Part model, mm, in its own coordinate system. A direction names the side the tool comes from. Round coordinates to 2 decimals unless told otherwise and drop trailing zeros. Write each loop counter-clockwise with the first axis right and the second up, starting at its lowest first coordinate (ties: lowest second). Pieces come first, ordered by that corner, then holes.
```python
from build123d import *

# Parameters (mm, degrees)
BOSS_EXTRUDE1_DEPTH = 18
SKETCH2_W           = 68
SKETCH2_H           = 20
CUT_EXTRUDE1_DEPTH  = 2
FILLET1_R           = 2
SKETCH3_W           = 20
SKETCH3_H           = 20
CUT_EXTRUDE4_DEPTH  = 7
SKETCH6_R           = 6.203606153
CUT_EXTRUDE5_DEPTH  = 103.004901843
CUT_EXTRUDE6_START  = -41
CUT_EXTRUDE6_DEPTH  = 41
FILLET2_R           = 6


# Read off the part's stored shape, not the designer's step: Cut-Extrude6
with BuildPart() as part:
    # Sketch1 → Boss-Extrude1 (new, symmetric)
    with BuildSketch(Plane.XY):
        with BuildLine():
            Line((-84, 0), (84, 0))
            Line((84, 0), (80, 14))
            Line((80, 14), (43, 14))
            Line((43, 14), (43, 55))
            Line((43, 55), (22, 55))
            Line((22, 55), (22, 43))
            Line((22, 43), (19, 43))
            Line((19, 43), (19, 40))
            ThreePointArc((19, 40), (0, 21), (-19, 40))
            Line((-19, 40), (-19, 43))
            Line((-19, 43), (-22, 43))
            Line((-22, 43), (-22, 55))
            Line((-22, 55), (-43, 55))
            Line((-43, 55), (-43, 14))
            Line((-43, 14), (-80, 14))
            Line((-80, 14), (-84, 0))
        make_face()
    extrude(amount=BOSS_EXTRUDE1_DEPTH, both=True)

    # Sketch2 → Cut-Extrude1 (cut)
    with BuildSketch(Plane.XZ):
        with Locations((-42, 0)):
            Rectangle(SKETCH2_W, SKETCH2_H)
        with Locations((42, 0)):
            Rectangle(SKETCH2_W, SKETCH2_H)
    extrude(amount=-CUT_EXTRUDE1_DEPTH, mode=Mode.SUBTRACT)

    # Fillet1
    fillet1_edges = [part.edges().sort_by_distance(p)[0] for p in [
        (76, 2, 0),
        (8, 2, 0),
        (-8, 2, 0),
        (-76, 2, 0),
    ]]
    fillet(fillet1_edges, radius=FILLET1_R - 0.0001)  # a hair under: the kernel refuses the full size

    # Sketch3 → Cut-Extrude4 (cut)
    with BuildSketch(Plane.XZ):
        with Locations((-31, 0)):
            Rectangle(SKETCH3_W, SKETCH3_H)
        with Locations((31, 0)):
            Rectangle(SKETCH3_W, SKETCH3_H)
    extrude(amount=-CUT_EXTRUDE4_DEPTH, mode=Mode.SUBTRACT)

    # Sketch6 → Cut-Extrude5 (cut, through all)
    with BuildSketch(Plane.XZ):
        with Locations(Location((-31, 0, 0), (0, 0, 270))):
            Circle(SKETCH6_R)
        with Locations(Location((31, 0, 0), (0, 0, 90))):
            Circle(SKETCH6_R)
        with BuildLine():
            Line((-68, 5), (-60, 5))
            ThreePointArc((-60, 5), (-55, 0), (-60, -5))
            Line((-60, -5), (-68, -5))
            ThreePointArc((-68, -5), (-73, 0), (-68, 5))
        make_face()
        with BuildLine():
            Line((68, 5), (60, 5))
            ThreePointArc((60, 5), (55, 0), (60, -5))
            Line((60, -5), (68, -5))
            ThreePointArc((68, -5), (73, 0), (68, 5))
        make_face()
    extrude(amount=-CUT_EXTRUDE5_DEPTH, mode=Mode.SUBTRACT)

    # Cut-Extrude6 outline → Cut-Extrude6 (cut)
    with BuildSketch(Plane(origin=(0, 55, 0), x_dir=(1, 0, 0), z_dir=(0, 1, 0)).offset(CUT_EXTRUDE6_START)):
        with BuildLine():
            ThreePointArc((43, 0), (42.001212365, -9.214019744), (39.05124838, -18))
            Line((39.05124838, -18), (43, -18))
            Line((43, -18), (43, 0))
        make_face()
        with BuildLine():
            ThreePointArc((39.05124838, 18), (42.001212365, 9.214019744), (43, 0))
            Line((43, 0), (43, 18))
            Line((43, 18), (39.05124838, 18))
        make_face()
        with BuildLine():
            Line((-43, -18), (-39.05124838, -18))
            ThreePointArc((-39.05124838, -18), (-42.001212365, -9.214019744), (-43, 0))
            Line((-43, 0), (-43, -18))
        make_face()
        with BuildLine():
            Line((-43, 18), (-43, 0))
            ThreePointArc((-43, 0), (-42.001212365, 9.214019744), (-39.05124838, 18))
            Line((-39.05124838, 18), (-43, 18))
        make_face()
    extrude(amount=CUT_EXTRUDE6_DEPTH, mode=Mode.SUBTRACT)

    # Fillet2
    fillet2_edges = [part.edges().sort_by_distance(p)[0] for p in [
        (42.001212365, 14, -9.214019744),
        (-42.001212365, 14, 9.214019744),
    ]]
    fillet(fillet2_edges, radius=FILLET2_R)

    # Sketch8 → Cut-Revolve1 (revolve, cut)
    with BuildSketch(Plane.XY, mode=Mode.PRIVATE) as cut_revolve1_sk:
        Polygon((0, 21), (0, 13.435755104), (3, 15.238336961), (3, 21.238336961), align=None)
    revolve(cut_revolve1_sk.sketch.rotate(Axis((0, 21, 0), (0, -1, 0)), 180), axis=Axis((0, 21, 0), (0, -1, 0)), mode=Mode.SUBTRACT)


solid = part.part
```
Q1. Drop flat-ended pins along their axis: pin 1 (1 mm diameter, centred on x = 11.5, z = -12.5, fed in from +Y); pin 2 (4 mm diameter, centred on x = 35.5, z = -5, fed in from -Y); pin 3 (3.5 mm diameter, centred on x = -16, z = -2.5, fed in from -Y). Give the stop position or say it passes through.
Values follow:
pin 1: stops at y = 25.27
pin 2: stops at y = 7
pin 3: stops at y = 2
Q2. Mould opens along X. For faces 5 (the flat face through (-1, 0, 0)), 6 (the flat face through (64, 8, -5)), 7 (the flat face through (22, 49, 0)) say: +X half, -X half, draft (parallel to the pull), parting line (faces both ways), or undercut.
Values follow:
face 5: draft
face 6: undercut
face 7: undercut
Q3. Wall check: L1, parallel to X at y = 44, z = 0; L2, parallel to Z at x = 0, y = 17; L3, parallel to X at y = 3.5, z = -4.5. Give the ranges that are in metal, low to high.
Values follow:
L1: x = -43 to -37.2, -24.8 to -22, 22 to 24.8, 37.2 to 43
L2: z = -18 to -3, 3 to 18
L3: x = -83 to -70.18, -57.82 to -41, -21 to 21, 41 to 57.82, 70.18 to 83
Q4. Which spindle directions (+Z, -Z, +X, -X, +Y, -Y) get a long thin tool onto all of the face, cutting with end or side? Do faces 1 (the flat face through (-42, 1, 10)), 2 (the conical face through (0.11, 13.75, 0.51)), 3 (the flat face through (-64, 8, -5)), 4 (the flat face through (-22, 49, 0)). Say none if no direction does.
Values follow:
face 1: -Y
face 2: +Y
face 3: +Y, -Y
face 4: +Z, -Z, +Y
Q5. Cut at A-A on y = 50.5. Write the cut outline in (x, z), plus the area to 3 significant figures.
Values follow:
outline: (-39.05, -18) - (-22, -18) - (-22, 18) - (-39.05, 18) arc R43 ccw to start; (22, -18) - (39.05, -18) arc R43 ccw to (39.05, 18) - (22, 18) - close; hole circle Ø12.41 at (-31, 0); hole circle Ø12.41 at (31, 0)
area: 1,180 mm2
Q6. Cut at D-D on y = 5.5. Write the cut outline in (x, z).
Values follow:
outline: (-82.43, -18) - (82.43, -18) - (82.43, 18) - (-82.43, 18) - close; hole (-68, -5) - (-60, -5) arc R5 ccw to (-60, 5) - (-68, 5) arc R5 ccw to start; hole (-41, -10) - (-21, -10) - (-21, 10) - (-41, 10) - close; hole (21, -10) - (41, -10) - (41, 10) - (21, 10) - close; hole (60, -5) - (68, -5) arc R5 ccw to (68, 5) - (60, 5) arc R5 ccw to start
Q7. Cut at C-C on y = 17. Write the cut outline in (x, z).
Values follow:
outline: (-39.93, -18) - (39.93, -18) arc R43.8 ccw to (39.93, 18) - (-39.93, 18) arc R43.8 ccw to start; hole circle Ø12.41 at (-31, 0); hole circle Ø6 at (0, 0); hole circle Ø12.41 at (31, 0)
Q8. Cut at B-B on x = -62. Write the cut outline in (y, z).
Values follow:
outline: (0, -18) - (14, -18) - (14, -5) - (2, -5) - (2, -10) - (0, -10) - close; (0, 10) - (2, 10) - (2, 5) - (14, 5) - (14, 18) - (0, 18) - close
